```python
from build123d import *

# Parameters (mm, degrees)
BOSS_EXTRUDE1_DEPTH       = 508
TAP_DRILL_FOR_4_12_TAP1_D = 99.6569
SKETCH8_W                 = 1016
SKETCH8_H                 = 508
CUT_EXTRUDE1_DEPTH        = 254
FILLET1_R                 = 177.8
CHAMFER1_SIZE             = 25.4


with BuildPart() as part:
    # Sketch3 → Boss-Extrude1 (new body)
    with BuildSketch(Plane.XY):
        with BuildLine():
            Line((2286, 762), (2540, 762))
            Line((2540, 762), (2286, 1016))
            Line((2286, 1016), (0, 1016))
            Line((0, 1016), (0, 0))
            ThreePointArc((0, 0), (254, -254), (508, 0))
            Line((508, 0), (2286, 0))
            Line((2286, 0), (2286, 762))
        make_face()
    extrude(amount=BOSS_EXTRUDE1_DEPTH)

    # Tap Drill for 4-12 Tap1 (through all)
    with Locations(Plane(origin=(254, 0, 508), x_dir=(1, 0, 0), z_dir=(0, 0, 1))):
        with Locations((0, 0)):
            Hole(TAP_DRILL_FOR_4_12_TAP1_D / 2)

    # Sketch8 → Cut-Extrude1 (cut)
    with BuildSketch(Plane.XY.offset(508)):
        with Locations((1143, 508)):
            Rectangle(SKETCH8_W, SKETCH8_H)
    extrude(amount=-CUT_EXTRUDE1_DEPTH, mode=Mode.SUBTRACT)

    # Fillet1
    fillet1_edges = [part.edges().sort_by_distance(p)[0] for p in [
        (2286, 0, 254),
    ]]
    fillet(fillet1_edges, radius=FILLET1_R)

    # Chamfer1
    chamfer1_edges = [part.edges().sort_by_distance(p)[0] for p in [
        (2286, 469.9, 508),
        (2233.923585695, 52.076414305, 508),
        (1308.1, 0, 508),
    ]]
    chamfer(chamfer1_edges, length=CHAMFER1_SIZE)


solid = part.part
```
Model file for the job. Use its own axes, mm. A direction names the side the tool comes from. Coordinates: 2 decimals unless noted, no trailing zeros. Order: outer loops, then holes, each group sorted by start corner. A loop starts at its lowest first (then second) coordinate and runs counter-clockwise, first axis right, second up. Notation, with made-up numbers: (58.5, 69.5) -> (63.5, 69.5) arc R35 ccw to (63.5, 105.5) -> close; hole circle Ø2 at (60, 46.5). An arc over 180 degrees is marked (long way). Return JSON: item names as keys, results as strings.
Item 1: Slice it at D-D (y = 205.5). Write the cut outline in (x, z), then the cut area to 3 significant figures.
Model answer:
{"outline": "(0, 0) -> (2286, 0) -> (2286, 482.6) -> (2260.6, 508) -> (0, 508) -> close", "area": "1,160,000 mm²"}
Item 2: Wall check: line 1 along Y through (x, z) = (254, 155); line 2 along X through (y, z) = (-21, 109); line 3 along Y through (x, z) = (984.5, 144.5). Give the ranges that are in metal, low to high. Write a range as from..to.
Model answer:
{"line 1": "y = -254..-49.83, 49.83..1016", "line 2": "x = 0.87..208.81, 299.19..507.13", "line 3": "y = 0..1016"}
Item 3: Slice it at B-B (z = 456.5). Write the cut outline in (x, y).
Model answer:
{"outline": "(0, 0) arc R254 ccw to (508, 0) -> (2108.2, 0) arc R177.8 ccw to (2286, 177.8) -> (2286, 762) -> (2540, 762) -> (2286, 1016) -> (0, 1016) -> close; hole circle Ø99.66 at (254, 0); hole (635, 254) -> (1651, 254) -> (1651, 762) -> (635, 762) -> close"}
Item 4: Pin check, flat tips, straight feed: P1, Ø5, axis at y = 207.5, z = 119.5, coming from the +X side; P2, Ø2, axis at x = 1539.5, z = 191.5, coming from the -Y side. Stop position of each tip, or through.
Model answer:
{"P1": "stops at x = 2286", "P2": "stops at y = 0"}
Item 5: Mould opens along X. For faces 4 (the face through (2286, 466, 238)), 5 (the face through (1136, 254, 383)), 6 (the face through (970, 249, 508)) say: pulls with the +X half, pulls with the -X half, needs draft (parallel to the pull), parting line crosses it, or undercut.
Model answer:
{"face 4": "pulls with the +X half", "face 5": "undercut", "face 6": "needs draft"}
Item 6: Slice it at C-C (z = 73.5). Write the cut outline in (x, y).
Model answer:
{"outline": "(0, 0) arc R254 ccw to (508, 0) -> (2108.2, 0) arc R177.8 ccw to (2286, 177.8) -> (2286, 762) -> (2540, 762) -> (2286, 1016) -> (0, 1016) -> close; hole circle Ø99.66 at (254, 0)"}
Item 7: 3-axis set-ups, long thin cutter, end or side, ignore diameter. For faces 1 (the face through (1136, 762, 383)), 2 (the face through (206.473, 14.967, 250.444)), 3 (the face through (1297, 0, 238)): which of +Z, -Z, +X, -X, +Y, -Y reach the whole face in a straight line?
Model answer:
{"face 1": "+Z", "face 2": "+Z, -Z", "face 3": "+Z, -Z, +X, -Y"}
Item 8: Slice it at A-A (x = 254). Write the cut outline in (y, z).
Model answer:
{"outline": "(-254, 0) -> (-49.83, 0) -> (-49.83, 508) -> (-254, 508) -> close; (49.83, 0) -> (1016, 0) -> (1016, 508) -> (49.83, 508) -> close"}
